Check sheet for the modelled part. Datum: model origin and axes. Units: mm. A direction names the side the tool comes from. Give positions to 0.01 mm unless a question says otherwise; leave off trailing zeros. Order: outer loops, then holes, each group sorted by start corner. A loop starts at its lowest first (then second) coordinate and runs counter-clockwise, first axis right, second up. Notation, with made-up numbers: M 50,77.25 L 93,77.25 A16 cw 93,82.25 Z; hole C 65,25 d1. An arc over 180 degrees is marked long. Answer in a Markdown table with one row per item. Add a question column.
from build123d import *

# Parameters (mm, degrees)
SKETCH1_R           = 3
BOSS_EXTRUDE2_DEPTH = 3
SKETCH4_R           = 1.25
SKETCH4_R_2         = 8.5
CUT_EXTRUDE2_DEPTH  = 10


with BuildPart() as part:
    # Sketch1 → Boss-Extrude2 (new body)
    with BuildSketch(Plane.XY):
        with BuildLine():
            Line((-34.17966517, 1.656542757), (-34.17966517, 41.656542757))
            Line((-34.17966517, 41.656542757), (-64.17966517, 41.656542757))
            Line((-64.17966517, 41.656542757), (-64.17966517, -38.343457243))
            ThreePointArc((-64.17966517, -38.343457243), (0.82033483, -53.158398897), (65.82033483, -38.343457243))
            Line((65.82033483, -38.343457243), (65.82033483, 41.656542757))
            Line((65.82033483, 41.656542757), (35.82033483, 41.656542757))
            Line((35.82033483, 41.656542757), (35.82033483, 1.656542757))
            ThreePointArc((35.82033483, 1.656542757), (0.82033483, -7.721678978), (-34.17966517, 1.656542757))
        make_face()
        with Locations((56.82033483, 20.554474708)):
            Circle(SKETCH1_R, mode=Mode.SUBTRACT)
        with Locations((42.82033483, 20.554474708)):
            Circle(SKETCH1_R, mode=Mode.SUBTRACT)
        with Locations((-55.17966517, 20.554474708)):
            Circle(SKETCH1_R, mode=Mode.SUBTRACT)
        with Locations((-41.17966517, 20.554474708)):
            Circle(SKETCH1_R, mode=Mode.SUBTRACT)
    extrude(amount=BOSS_EXTRUDE2_DEPTH)

    # Sketch4 → Cut-Extrude2 (cut)
    with BuildSketch(Plane.XY.offset(3)):
        with Locations((7.78, -22.696934593)):
            Circle(SKETCH4_R)
        with Locations((7.78, -38.256934593)):
            Circle(SKETCH4_R)
        with Locations((-7.78, -38.256934593)):
            Circle(SKETCH4_R)
        with Locations((-7.78, -22.696934593)):
            Circle(SKETCH4_R)
        with Locations((0, -30.476934593)):
            Circle(SKETCH4_R_2)
    extrude(amount=-CUT_EXTRUDE2_DEPTH, mode=Mode.SUBTRACT)


solid = part.part
Q1. Tool access check on faces 1 (the flat face through (-34.18, 21, 1)), 2 (the cylindrical face through (39.823, 20.686, 1.479)). Record the directions out of +Z, -Z, +X, -X, +Y, -Y that give a thin tool (end or side, any length) a straight path to the whole face; none if there is none.
Q2. Cross-section at B-B (z = 0.55). State how many separate pieces and enclosed holes the cut face has, and give its area (3 significant figures).
Q3. Cross-section at A-A (y = 25.5). Record the boundary of the cut face in (x, z), and give its area (3 significant figures).
Q4. Cross-section at C-C (x = 0). Record the boundary of the cut face in (y, z).
Q5. Cross-section at D-D (x = -26). Record the boundary of the cut face in (y, z).
Q6. Thickness scan on probe 1 along Y at (x, z) = (-7.78, 2.25); probe 2 along X at (y, z) = (7, 1.55); probe 3 along X at (y, z) = (21, 2.8). Record the ranges inside material, lowest first.
Q7. Draft check along Y on faces 3 (the cylindrical face through (-58.177, 20.686, 1.479)), 4 (the cylindrical face through (-0.121, -53.155, 1.479)), 5 (the flat face through (35.82, 22, 1)). Enter one of: pulls with the +Y half, pulls with the -Y half, needs draft (parallel to the pull), parting line crosses it, or undercut.
Values follow:
| question | item | result |
|---|---|---|
| 1 | face 1 | +Z, -Z, +Y |
| 1 | face 2 | +Z, -Z |
| 2 | separate pieces | 1 |
| 2 | enclosed holes | 9 |
| 2 | area | 8,090 mm² |
| 3 | outline | M -64.18,0 L -34.18,0 L -34.18,3 L -64.18,3 Z; M 35.82,0 L 65.82,0 L 65.82,3 L 35.82,3 Z |
| 3 | area | 180 mm² |
| 4 | outline | M -53.16,0 L -38.98,0 L -38.98,3 L -53.16,3 Z; M -21.98,0 L -7.72,0 L -7.72,3 L -21.98,3 Z |
| 5 | outline | M -50.74,0 L -2.38,0 L -2.38,3 L -50.74,3 Z |
| 6 | probe 1 | -52.91 to -39.51, -37.01 to -33.9, -27.05 to -23.95, -21.45 to -7.19 |
| 6 | probe 2 | -64.18 to -34.18, 35.82 to 65.82 |
| 6 | probe 3 | -64.18 to -58.15, -52.21 to -44.15, -38.21 to -34.18, 35.82 to 39.85, 45.79 to 53.85, 59.79 to 65.82 |
| 7 | face 3 | undercut |
| 7 | face 4 | pulls with the -Y half |
| 7 | face 5 | needs draft |
